Geometry: final body of the model. Coordinates: model frame, mm. Face numbers are marked on the shaded views. A direction names the side the tool comes from. Give positions to 0.01 mm unless a question says otherwise; leave off trailing zeros. Write each loop counter-clockwise with the first axis right and the second up, starting at its lowest first coordinate (ties: lowest second). Pieces come first, ordered by that corner, then holes. Notation, with made-up numbers: (-26.75, 80.25) -> (2.25, 80.25) arc R28 ccw to (2.25, 103.25) -> close; hole circle Ø2 at (-1.5, 82.5). An arc over 180 degrees is marked (long way). Answer as a JSON object with one key per item and string values. Group by question number.
(1) Contact query for flat-ended pins moving along their axis: pin 1 Ø3.5 at (x, z) = (10.5, -10) entering from +Y; pin 2 Ø0.8 at (x, z) = (17.5, -14.5) entering from +Y; pin 3 Ø4.5 at (x, y) = (9.74, -15.5) entering from -Z; pin 4 Ø0.9 at (y, z) = (52.5, -8.5) entering from +X. Output: stop coordinate, or through.
(2) Section query B-B on y = 60.5. Output: boundary loops of the cut face in (x, z), plus the area to 3 significant figures.
(3) Material intervals for probe 1 along Z at (x, y) = (-19, 7.5); probe 2 along X at (y, z) = (20, -7.5); probe 3 along Y at (x, z) = (-16, -5.25), sorted ascending.
(4) Section query A-A on x = 7.5. Output: boundary loops of the cut face in (y, z), plus the area to 3 significant figures.
(5) Section query C-C on x = -15.5. Output: boundary loops of the cut face in (y, z), plus the area to 3 significant figures.
(6) Section query D-D on z = -11. Output: boundary loops of the cut face in (x, y).
(7) Draft query along X for the marked faces 1, 2 and 3. Return one class per face: +X half, -X half, draft (parallel to the pull), parting line (faces both ways), or undercut.
(8) Set-up query: the marked faces 4, 5, 6 and 7. Return all of +Z, -Z, +X, -X, +Y, -Y with unobstructed straight access to the full face (end or side cutting, diameter ignored); none if empty.
from build123d import *

# Parameters (mm, degrees)
SKETCH1_R                      = 1.35
BASE_FLANGE1_DEPTH             = 0.8
EDGE_FLANGE1_STRIP_W           = 7.2
EDGE_FLANGE1_STRIP_H           = 0.8
EDGE_FLANGE1_STRIP_CUT_DEPTH   = 50
EDGE_FLANGE1_STRIP_2_W         = 7.2
EDGE_FLANGE1_STRIP_2_H         = 0.8
EDGE_FLANGE1_STRIP_CUT_2_DEPTH = 57
EDGE_FLANGE1_DEPTH             = 50
EDGE_FLANGE1_BEND_DEPTH        = 57
EDGE_FLANGE4_DEPTH             = 11.5
EDGE_FLANGE4_BEND_DEPTH        = 11.5
EDGE_FLANGE5_DEPTH             = 50
EDGE_FLANGE5_BEND_DEPTH        = 57


# Sheet-metal steps are written as plain solids
with BuildPart() as part:
    # Sketch1 → Base-Flange1 (new body)
    with BuildSketch(Plane.XY):
        Polygon((16.25, 0), (16.25, -18.5), (-14.25, -18.5), (-14.25, -7), (-23.25, -7), (-23.25, 50), (-14.25, 50), (-14.25, 63.5), (16.25, 63.5), (16.25, 50), (21.25, 50), (21.25, 0), align=None)
        with Locations((9.737756115, -15.5)):
            Circle(SKETCH1_R, mode=Mode.SUBTRACT)
        with Locations((-4.262243885, -15.5)):
            Circle(SKETCH1_R, mode=Mode.SUBTRACT)
        with Locations((9.737756115, 60.5)):
            Circle(SKETCH1_R, mode=Mode.SUBTRACT)
        with Locations((-4.262243885, 60.5)):
            Circle(SKETCH1_R, mode=Mode.SUBTRACT)
    extrude(amount=BASE_FLANGE1_DEPTH)

    # Edge-Flange1 strip (across the edge) → Edge-Flange1 strip cut (cut)
    with BuildSketch(Plane(origin=(21.25, 50, 0), x_dir=(-1, 0, 0), z_dir=(0, -1, 0))):
        with Locations((-1.6, -0.4)):
            Rectangle(EDGE_FLANGE1_STRIP_W, EDGE_FLANGE1_STRIP_H)
    extrude(amount=EDGE_FLANGE1_STRIP_CUT_DEPTH, mode=Mode.SUBTRACT)

    # Edge-Flange1 strip 2 (across the edge) → Edge-Flange1 strip cut 2 (cut)
    with BuildSketch(Plane(origin=(-23.25, -7, 0), x_dir=(1, 0, 0), z_dir=(0, 1, 0))):
        with Locations((-1.6, -0.4)):
            Rectangle(EDGE_FLANGE1_STRIP_2_W, EDGE_FLANGE1_STRIP_2_H)
    extrude(amount=EDGE_FLANGE1_STRIP_CUT_2_DEPTH, mode=Mode.SUBTRACT)

    # Edge-Flange1 section (across the edge) → Edge-Flange1 (add)
    with BuildSketch(Plane(origin=(21.25, 50, 0), x_dir=(-1, 0, 0), z_dir=(0, -1, 0))):
        with BuildLine():
            Line((-0.8, 2), (-0.8, 13.5))
            Line((-0.8, 13.5), (0, 13.5))
            Line((0, 13.5), (0, 2))
            ThreePointArc((0, 2), (0.585786438, 0.585786438), (2, 0))
            Line((2, 0), (2, -0.8))
            ThreePointArc((2, -0.8), (0.020101013, 0.020101013), (-0.8, 2))
        make_face()
    extrude(amount=EDGE_FLANGE1_DEPTH)

    # Edge-Flange1 section 2 (across the edge) → Edge-Flange1 bend (add)
    with BuildSketch(Plane(origin=(-23.25, -7, 0), x_dir=(1, 0, 0), z_dir=(0, 1, 0))):
        with BuildLine():
            Line((-0.8, 2), (-0.8, 13.5))
            Line((-0.8, 13.5), (0, 13.5))
            Line((0, 13.5), (0, 2))
            ThreePointArc((0, 2), (0.585786438, 0.585786438), (2, 0))
            Line((2, 0), (2, -0.8))
            ThreePointArc((2, -0.8), (0.020101013, 0.020101013), (-0.8, 2))
        make_face()
    extrude(amount=EDGE_FLANGE1_BEND_DEPTH)

    # Edge-Flange4 section (across the edge) → Edge-Flange4 (add)
    with BuildSketch(Plane(origin=(21.25, 52, -2), x_dir=(0, -1, 0), z_dir=(0, 0, -1))):
        with BuildLine():
            Line((-0.8, 2), (-0.8, 20))
            Line((-0.8, 20), (0, 20))
            Line((0, 20), (0, 2))
            ThreePointArc((0, 2), (0.585786438, 0.585786438), (2, 0))
            Line((2, 0), (2, -0.8))
            ThreePointArc((2, -0.8), (0.020101013, 0.020101013), (-0.8, 2))
        make_face()
    extrude(amount=EDGE_FLANGE4_DEPTH)

    # Edge-Flange4 section 2 (across the edge) → Edge-Flange4 bend (add)
    with BuildSketch(Plane(origin=(-23.25, 52, -13.5), x_dir=(0, -1, 0), z_dir=(0, 0, 1))):
        with BuildLine():
            Line((-0.8, 2), (-0.8, 20))
            Line((-0.8, 20), (0, 20))
            Line((0, 20), (0, 2))
            ThreePointArc((0, 2), (0.585786438, 0.585786438), (2, 0))
            Line((2, 0), (2, -0.8))
            ThreePointArc((2, -0.8), (0.020101013, 0.020101013), (-0.8, 2))
        make_face()
    extrude(amount=EDGE_FLANGE4_BEND_DEPTH)

    # Edge-Flange5 section (across the edge) → Edge-Flange5 (add)
    with BuildSketch(Plane(origin=(21.25, 50, -15.5), x_dir=(0, 0, 1), z_dir=(0, -1, 0))):
        with BuildLine():
            Line((-0.8, 2), (-0.8, 10))
            Line((-0.8, 10), (0, 10))
            Line((0, 10), (0, 2))
            ThreePointArc((0, 2), (0.585786438, 0.585786438), (2, 0))
            Line((2, 0), (2, -0.8))
            ThreePointArc((2, -0.8), (0.020101013, 0.020101013), (-0.8, 2))
        make_face()
    extrude(amount=EDGE_FLANGE5_DEPTH)

    # Edge-Flange5 section 2 (across the edge) → Edge-Flange5 bend (add)
    with BuildSketch(Plane(origin=(-23.25, -7, -15.5), x_dir=(0, 0, 1), z_dir=(0, 1, 0))):
        with BuildLine():
            Line((-0.8, 2), (-0.8, 10))
            Line((-0.8, 10), (0, 10))
            Line((0, 10), (0, 2))
            ThreePointArc((0, 2), (0.585786438, 0.585786438), (2, 0))
            Line((2, 0), (2, -0.8))
            ThreePointArc((2, -0.8), (0.020101013, 0.020101013), (-0.8, 2))
        make_face()
    extrude(amount=EDGE_FLANGE5_BEND_DEPTH)


solid = part.part
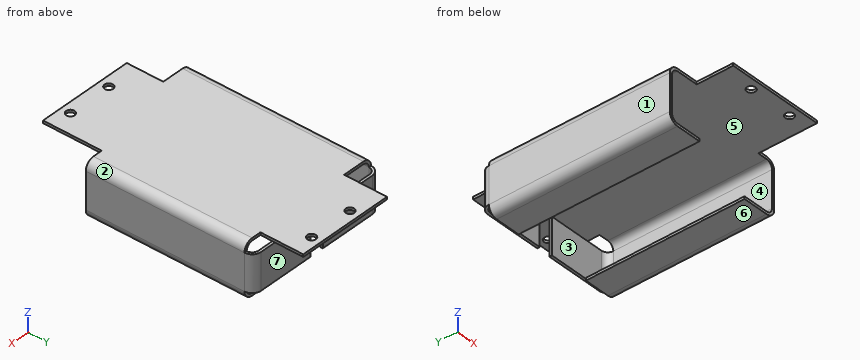
Answer list:
{
 "1": {"pin 1": "y = 52.8", "pin 2": "through", "pin 3": "z = 0", "pin 4": "x = 21.16"},
 "2": {"outline": "(-14.25, 0) -> (-5.61, 0) -> (-5.61, 0.8) -> (-14.25, 0.8) -> close; (-2.91, 0) -> (8.39, 0) -> (8.39, 0.8) -> (-2.91, 0.8) -> close; (11.09, 0) -> (16.25, 0) -> (16.25, 0.8) -> (11.09, 0.8) -> close", "area": "20.1 mm2"},
 "3": {"probe 1": "-16.3 to -15.5, 0 to 0.8", "probe 2": "-24.05 to -23.25, 21.25 to 22.05", "probe 3": "52 to 52.8"},
 "4": {"outline": "(-18.5, 0) -> (63.5, 0) -> (63.5, 0.8) -> (-18.5, 0.8) -> close; (52, -13.5) -> (52.8, -13.5) -> (52.8, -2) -> (52, -2) -> close", "area": "74.8 mm2"},
 "5": {"outline": "(-7, -16.3) -> (50, -16.3) -> (50, -15.5) -> (-7, -15.5) -> close; (-7, 0) -> (50, 0) -> (50, 0.8) -> (-7, 0.8) -> close; (52, -13.5) -> (52.8, -13.5) -> (52.8, -2) -> (52, -2) -> close", "area": "100 mm2"},
 "6": {"outline": "(-24.05, -7) -> (-23.25, -7) -> (-23.25, 50) arc R2 cw to (-21.25, 52) -> (-3.25, 52) -> (-3.25, 52.8) -> (-21.25, 52.8) arc R2.8 ccw to (-24.05, 50) -> close; (1.25, 52) -> (19.25, 52) arc R2 cw to (21.25, 50) -> (21.25, 0) -> (22.05, 0) -> (22.05, 50) arc R2.8 ccw to (19.25, 52.8) -> (1.25, 52.8) -> close"},
 "7": {"face 1": "-X half", "face 2": "+X half", "face 3": "undercut"},
 "8": {"face 4": "-Y", "face 5": "+Y, -Y", "face 6": "-Z, +X, -X, +Y, -Y", "face 7": "-Z, +X, -X, +Y"}
}
